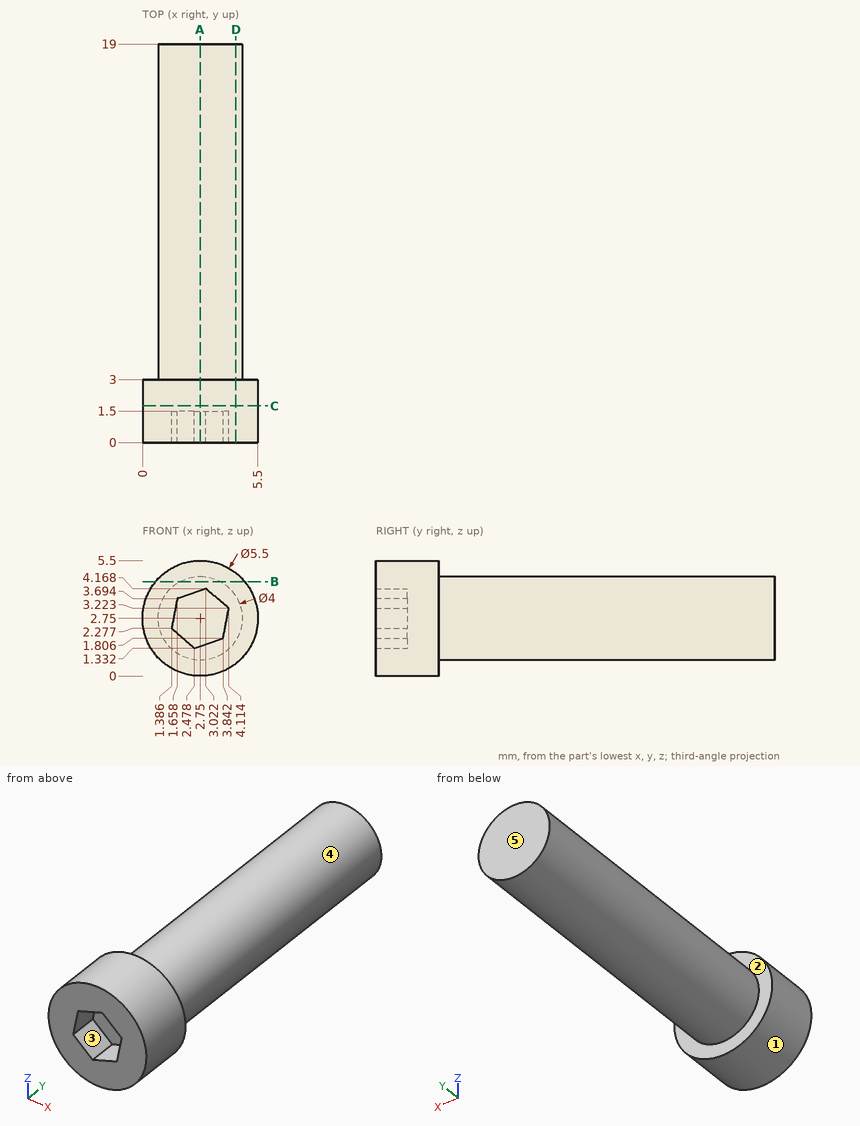
Design review of the part shown in the three views and the two pictorial views. Dimensions are in mm from the part's minimum x, y and z. A direction names the side the tool comes from. Round coordinates to 2 decimals unless told otherwise and drop trailing zeros. Write each loop counter-clockwise with the first axis right and the second up, starting at its lowest first coordinate (ties: lowest second). Pieces come first, ordered by that corner, then holes.
1) Machinability: for the marked faces 1 and 2, which of the approach directions +Z, -Z, +X, -X, +Y, -Y give a long, thin tool a straight path to every point of the face, cutting with its end or side? Answer none if there is none.
Answer below:
face 1: +Y, -Y
face 2: +Y
2) Take a section at C-C on y = 1.75. Give the boundary of the cut face in (x, z).
Answer below:
outline: circle Ø5.5 at (2.75, 2.75)
3) Mouldability with a two-part tool opening along Z and no side actions: class the marked faces 3, 4 and 5 as +Z half, -Z half, draft (parallel to the pull), parting line (faces both ways), or undercut.
Answer below:
face 3: undercut
face 4: parting line
face 5: draft
4) Insertion check: pin 1 Ø1.4 at (x, z) = (2.5, 2.5) entering from -Y; pin 2 Ø1.5 at (y, z) = (9.5, 2) entering from +X; pin 3 Ø1 at (y, z) = (12, 1.5) entering from -X (1 decimal). Each pin has a flat end and moves straight along its axis. Give the tip position at first contact, or say it passes through.
Answer below:
pin 1: stops at y = 1.5
pin 2: stops at x = 4.75
pin 3: stops at x = 0.9
5) Take a section at A-A on x = 2.75. Give the boundary of the cut face in (y, z).
Answer below:
outline: (0, 0) - (3, 0) - (3, 0.75) - (19, 0.75) - (19, 4.75) - (3, 4.75) - (3, 5.5) - (0, 5.5) - (0, 4.07) - (1.5, 4.07) - (1.5, 1.43) - (0, 1.43) - close
6) For line 1 along Y through (x, z) = (0.6, 2.55); line 2 along X through (y, z) = (11.25, 2.7); line 3 along X through (y, z) = (2, 1), list the stretches that pass through material, from the lowest coordinate up.
Answer below:
line 1: y = 0 to 3
line 2: x = 0.75 to 4.75
line 3: x = 0.63 to 4.87
7) Take a section at D-D on x = 4.45. Give the boundary of the cut face in (y, z).
Answer below:
outline: (0, 0.59) - (3, 0.59) - (3, 1.7) - (19, 1.7) - (19, 3.8) - (3, 3.8) - (3, 4.91) - (0, 4.91) - close
8) Take a section at B-B on z = 4.5. Give the boundary of the cut face in (x, y).
Answer below:
outline: (0.63, 0) - (4.87, 0) - (4.87, 3) - (3.72, 3) - (3.72, 19) - (1.78, 19) - (1.78, 3) - (0.63, 3) - close
